Check sheet for the modelled part. Datum: model origin and axes. Units: mm. A direction names the side the tool comes from. Coordinates: 2 decimals unless noted, no trailing zeros. Loops run counter-clockwise (first coordinate to the right, second up) from the corner with the lowest first, then second, coordinate; pieces in that order, holes last. Notation, with made-up numbers: (-24.5, 66) -> (23.5, 66) arc R29 ccw to (23.5, 92) -> close; hole circle Ø7 at (-25, 1). An arc over 180 degrees is marked (long way). Use one line per item in the form item = value.
from build123d import *

# Parameters (mm, degrees)
SKETCH1_W           = 50
SKETCH1_H           = 15
BOSS_EXTRUDE1_DEPTH = 3
SKETCH2_R           = 2
CUT_EXTRUDE1_DEPTH  = 3
CUT_EXTRUDE2_DEPTH  = 3


with BuildPart() as part:
    # Sketch1 → Boss-Extrude1 (new body)
    with BuildSketch(Plane.XY):
        Rectangle(SKETCH1_W, SKETCH1_H)
    extrude(amount=BOSS_EXTRUDE1_DEPTH)

    # Sketch2 → Cut-Extrude1 (cut)
    with BuildSketch(Plane.XY.offset(3)):
        with Locations((-20, 0)):
            Circle(SKETCH2_R)
    extrude(amount=-CUT_EXTRUDE1_DEPTH, mode=Mode.SUBTRACT)

    # Sketch3 → Cut-Extrude2 (cut)
    with BuildSketch(Plane.XY.offset(3)):
        with BuildLine():
            Line((5.969403334, 1.726719429), (17.226282515, 1.726719429))
            ThreePointArc((17.226282515, 1.726719429), (18.953001944, 0), (17.226282515, -1.726719429))
            Line((17.226282515, -1.726719429), (5.969403334, -1.726719429))
            ThreePointArc((5.969403334, -1.726719429), (4.242683906, 0), (5.969403334, 1.726719429))
        make_face()
    extrude(amount=-CUT_EXTRUDE2_DEPTH, mode=Mode.SUBTRACT)


solid = part.part
(1) Go/stop test with a flat-tipped pin: P1, Ø3.5, axis at x = -20, y = 0, coming from the -Z side. Record where the tip stops, or that it passes through.
Established:
P1 = through
(2) Tool access check on faces 5 (the flat face through (12, -1.727, 2)), 6 (the flat face through (0, 7.5, 1)). Record the directions out of +Z, -Z, +X, -X, +Y, -Y that give a thin tool (end or side, any length) a straight path to the whole face; none if there is none.
Established:
face_5 = +Z, -Z
face_6 = +Z, -Z, +X, -X, +Y
(3) Scan lines: line 1 along Y through (x, z) = (-20, 1.25); line 2 along X through (y, z) = (-1.5, 1.1); line 3 along X through (y, z) = (-1, 2.6). Record each from-to range of solid material in increasing order.
Established:
line_1 = -7.5 to -2, 2 to 7.5
line_2 = -25 to -21.32, -18.68 to 5.11, 18.08 to 25
line_3 = -25 to -21.73, -18.27 to 4.56, 18.63 to 25
(4) Section check A-A, the plane z = 1.25. Record the boundary of the cut face in (x, y).
Established:
outline = (-25, -7.5) -> (25, -7.5) -> (25, 7.5) -> (-25, 7.5) -> close; hole circle Ø4 at (-20, 0); hole (5.97, -1.73) -> (17.23, -1.73) arc R1.73 ccw to (17.23, 1.73) -> (5.97, 1.73) arc R1.73 ccw to start
(5) Mould release check, pull along X, two halves, no side actions. Record for faces 1 (the flat face through (25, 0, 1)), 2 (the flat face through (0, 0, 0)), 3 (the cylindrical face through (18.953, 0.038, 1.521)), 4 (the cylindrical face through (-21.6, -1.2, 1.5)): +X half, -X half, draft (parallel to the pull), parting line (faces both ways), or undercut.
Established:
face_1 = +X half
face_2 = draft
face_3 = undercut
face_4 = undercut
(6) Section check C-C, the plane x = -20. Record the boundary of the cut face in (y, z).
Established:
outline = (-7.5, 0) -> (-2, 0) -> (-2, 3) -> (-7.5, 3) -> close; (2, 0) -> (7.5, 0) -> (7.5, 3) -> (2, 3) -> close
(7) Section check B-B, the plane y = 0. Record the boundary of the cut face in (x, z).
Established:
outline = (-25, 0) -> (-22, 0) -> (-22, 3) -> (-25, 3) -> close; (-18, 0) -> (4.24, 0) -> (4.24, 3) -> (-18, 3) -> close; (18.95, 0) -> (25, 0) -> (25, 3) -> (18.95, 3) -> close
